Geometry: final body of the model. Coordinates: model frame, mm. Face numbers are marked on the shaded views. A direction names the side the tool comes from. Coordinates: 2 decimals unless noted, no trailing zeros. Loops run counter-clockwise (first coordinate to the right, second up) from the corner with the lowest first, then second, coordinate; pieces in that order, holes last. Notation, with made-up numbers: M 74,-24.75 L 79,-24.75 A16 ccw 79,-18.75 Z; hole C -8,39.5 d2. An arc over 180 degrees is marked long. Write each question's results on one line, items separated by ' | '. Start each with the question number.
from build123d import *

# Parameters (mm, degrees)
SKETCH_1_R      = 1
EXTRUDE_1_DEPTH = 3
EXTRUDE_2_DEPTH = 3
FILLET_2_R      = 1
FILLET_3_R      = 1
EXTRUDE_4_DEPTH = 1


with BuildPart() as part:
    # 草图1 → 凸台-拉伸1 (new body)
    with BuildSketch(Plane.XY):
        with BuildLine():
            Line((-5, 0), (-5, -20))
            Line((-5, -20), (5, -20))
            Line((5, -20), (5, 0))
            ThreePointArc((5, 0), (0, 5), (-5, 0))
        make_face()
        Circle(SKETCH_1_R, mode=Mode.SUBTRACT)
    extrude(amount=EXTRUDE_1_DEPTH)

    # 草图2 → 凸台-拉伸2 (add)
    with BuildSketch(Plane.XY.offset(3)):
        Polygon((5, -20), (-5, -20), (-16.053330201, -28.571505672), (5, -28.571505672), align=None)
    extrude(amount=-EXTRUDE_2_DEPTH)

    # 圆角2
    fillet_2_edges = [part.edges().sort_by_distance(p)[0] for p in [
        (-16.053330201, -28.571505672, 1.5),
    ]]
    fillet(fillet_2_edges, radius=FILLET_2_R)

    # 圆角3
    fillet_3_edges = [part.edges().sort_by_distance(p)[0] for p in [
        (5, -28.571505672, 1.5),
    ]]
    fillet(fillet_3_edges, radius=FILLET_3_R)

    # 草图4 → 凸台-拉伸4 (add)
    with BuildSketch(Plane(origin=(0, 0, 0), x_dir=(-1, 0, 0), z_dir=(0, 0, -1))):
        Polygon((-4.275312121, -2.510402489), (-4.275312121, -12.516814932), (-2.995953453, -12.516814932), (-2.995953453, -8.633047546), (1.938715697, -12.516814932), (4.31466751, -12.516814932), (-2.995953453, -6.763085471), (4.31466751, -2.510402489), (1.207653601, -2.510402489), (-2.995953453, -4.955695204), (-2.995953453, -2.510402489), align=None)
        Polygon((-4.275312121, -15.401899276), (-4.275312121, -26.544068904), (-2.995953453, -26.544068904), (-2.995953453, -22.614610137), (1.938715697, -26.544068904), (4.31466751, -26.544068904), (-2.995953453, -20.722648508), (4.31466751, -15.401899276), (1.207653601, -15.401899276), (-2.995953453, -18.461330084), (-2.995953453, -15.401899276), align=None)
    extrude(amount=EXTRUDE_4_DEPTH)


solid = part.part
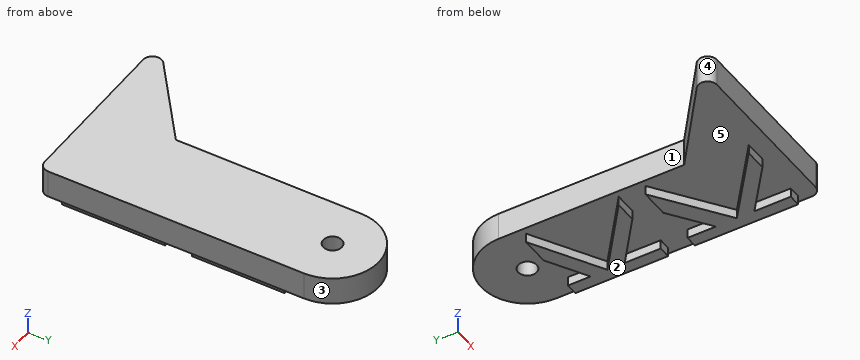
Item 1: Section D-D, the plane y = -12. Return loops of the section in (x, z), plus the area to 3 significant figures.
Item 2: Section C-C, the plane x = 0. Return loops of the section in (y, z), plus the area to 3 significant figures.
Item 3: Contact query for flat-ended pins moving along their axis: P1, Ø2.5, axis at x = 0, y = 0, coming from the -Z side; P2, Ø1, axis at x = -3, z = 2, coming from the +Y side; P3, Ø0.8, axis at x = 3.5, z = -0.5, coming from the -Y side. Output: stop coordinate, or through.
Item 4: Set-up query: the marked faces 1 and 2. Return all of +Z, -Z, +X, -X, +Y, -Y with unobstructed straight access to the full face (end or side cutting, diameter ignored); none if empty.
Item 5: Pull-direction query (X, two-part tool) for the marked faces 3, 4 and 5; classes: released by +X, released by -X, zero draft, split by the parting line, or undercut.
Item 6: Section A-A, the plane z = -0.5. Return loops of the section in (x, y).
Item 7: Ray query, L1, parallel to Y at x = 0.5, z = -0.2; L2, parallel to X at y = -5.5, z = 0.95; L3, parallel to Z at x = -1, y = -26. Return the intervals inside material, ascending. Write a range as [from, to].
Item 8: Section B-B, the plane z = 1.95. Return loops of the section in (x, y).
Solutions:
1) outline: M -5,0 L -3.66,0 L -3.66,-1 L -1.28,-1 L -1.28,0 L 3,0 L 3,-1 L 4.28,-1 L 4.28,0 L 5,0 L 5,3 L -5,3 Z | area: 33.7 mm²
2) outline: M -28.57,0 L -25,0 L -25,-1 L -23.11,-1 L -23.11,0 L -18.54,0 L -18.54,-1 L -16.28,-1 L -16.28,0 L -10.99,0 L -10.99,-1 L -9.12,-1 L -9.12,0 L -5.02,0 L -5.02,-1 L -3.21,-1 L -3.21,0 L -1,0 L -1,3 L -28.57,3 Z; M 1,0 L 5,0 L 5,3 L 1,3 Z | area: 103 mm²
3) P1: stops at z = 0 | P2: stops at y = 4.33 | P3: stops at y = -26.54
4) face 1: +Z, -Z, -X, +Y | face 2: -Z, +X, -X, +Y, -Y
5) face 3: split by the parting line | face 4: released by -X | face 5: undercut
6) outline: M -4.31,-26.54 L -1.94,-26.54 L 3,-22.61 L 3,-26.54 L 4.28,-26.54 L 4.28,-15.4 L 3,-15.4 L 3,-18.46 L -1.21,-15.4 L -4.31,-15.4 L 3,-20.72 Z; M -4.31,-12.52 L -1.94,-12.52 L 3,-8.63 L 3,-12.52 L 4.28,-12.52 L 4.28,-2.51 L 3,-2.51 L 3,-4.96 L -1.21,-2.51 L -4.31,-2.51 L 3,-6.76 Z
7) L1: y = [-24.6, -22.71], [-18.91, -16.64], [-10.6, -8.73], [-5.31, -3.5] | L2: x = [-5, 5] | L3: z = [0, 3]
8) outline: M -13.74,-26.78 A1 ccw -13.13,-28.57 L 4,-28.57 A1 ccw 5,-27.57 L 5,0 A5 ccw -5,0 L -5,-20 Z; hole C 0,0 d2
